Here's how the part is built. I have some questions about the finished solid (model axes, mm). A direction names the side the tool comes from. Coordinates: 2 decimals unless noted, no trailing zeros. Write each loop counter-clockwise with the first axis right and the second up, starting at its lowest first coordinate (ties: lowest second). Pieces come first, ordered by that corner, then holes. Notation, with made-up numbers: (25, 59) -> (33, 59) arc R24 cw to (33, 96) -> close; hole circle Ø11 at (57, -20.75). An arc over 180 degrees is marked (long way). Put each result on its own line as item: value. Start each with the question number.
Item 1: I need wall thicknesses on line 1 (Y direction, x = -11.5, z = 7); line 2 (X direction, y = -11.5, z = 4.5). Which ranges of each line are inside material? Lowest first, please. Write a range as [from, to].
Item 2: I want a section at A-A, the plane z = 9. List the corners of the cut face in (x, y) for me, then the cut area to 4 significant figures.
Item 3: I want a section at B-B, the plane x = 9.5. List the corners of the cut face in (y, z) for me.
Item 4: On a 3-axis mill with a long thin cutter (end or side, diameter ignored), from which of +Z, -Z, +X, -X, +Y, -Y can I reach the whole of each face in a straight line? I mean faces 1 (the face through (15.5, 11.5, 4.2)), 2 (the face through (0, 14, 1)), 3 (the face through (0, -14, 1)). Say none if no direction works.
Item 5: I want a section at C-C, the plane y = 11.5. List the corners of the cut face in (x, z) for me, then the cut area to 3 significant figures.
Item 6: For pin 1 (1.8 mm diameter, centred on x = -0.5, y = 15, fed in from +Z); pin 2 (2.5 mm diameter, centred on x = -5.5, z = 3, fed in from +Y); pin 3 (4 mm diameter, centred on x = 3, z = 1.5, fed in from +Y), each with a flat end and sliding along its axis, tell me the tip position at first contact or that it passes through.
Item 7: I want a section at D-D, the plane x = -5. List the corners of the cut face in (y, z) for me.
from build123d import *

# Parameters (mm, degrees)
F0_W        = 5
F0_H        = 6
F1_DEPTH    = 9.5
F2_DEPTH    = 1
F3_T1_DEPTH = 1
F3_T3_DEPTH = 16
F4_SIZE     = 1


# Not quite as in the source:
# - a fillet or chamfer that OpenCascade refuses, or shapes differently, is made with other operations: its cross-section is extruded or revolved along the edge and cut away or added


with BuildPart() as f1:
    # F0 (on Top) → F1 (new body)
    with BuildSketch(Plane.XY):
        Polygon((16, -12), (16, 12), (2.5, 12), (2.5, 6), (-2.5, 6), (-2.5, 12), (-16, 12), (-16, -12), (-2.5, -12), (-2.5, -6), (2.5, -6), (2.5, -12), align=None)
        with Locations((0, -9)):
            Rectangle(F0_W, F0_H)
        with Locations((0, 9)):
            Rectangle(F0_W, F0_H)
    extrude(amount=F1_DEPTH)

    # F0 (on Top) → F2 (join)
    with BuildSketch(Plane.XY):
        with Locations((0, 15)):
            Rectangle(F0_W, F0_H)
        with Locations((0, -15)):
            Rectangle(F0_W, F0_H)
    extrude(amount=F2_DEPTH)

    # F3: fillet of radius 3 on 8 edges, made by hand

    # F3_s2 → F3_t1 (join)
    with BuildSketch(Plane.XY):
        with BuildLine():
            ThreePointArc((5.5, -12), (3.3786796564, -12.8786796564), (2.5, -15))
            Line((2.5, -15), (2.5, -12))
            Line((2.5, -12), (5.5, -12))
        make_face()
        with BuildLine():
            ThreePointArc((-5.5, -12), (-3.3786796564, -12.8786796564), (-2.5, -15))
            Line((-2.5, -15), (-2.5, -12))
            Line((-2.5, -12), (-5.5, -12))
        make_face()
        with BuildLine():
            ThreePointArc((-5.5, 12), (-3.3786796564, 12.8786796564), (-2.5, 15))
            Line((-2.5, 15), (-2.5, 12))
            Line((-2.5, 12), (-5.5, 12))
        make_face()
        with BuildLine():
            ThreePointArc((5.5, 12), (3.3786796564, 12.8786796564), (2.5, 15))
            Line((2.5, 15), (2.5, 12))
            Line((2.5, 12), (5.5, 12))
        make_face()
    extrude(amount=F3_T1_DEPTH)

    # F3_s4 → F3_t3 (cut)
    with BuildSketch(Plane.XY.offset(-7.5)):
        with BuildLine():
            ThreePointArc((0.5, -18), (-1.6213203436, -17.1213203436), (-2.5, -15))
            Line((-2.5, -15), (-2.5, -18))
            Line((-2.5, -18), (0.5, -18))
        make_face()
        with BuildLine():
            ThreePointArc((2.5, -15), (1.6213203436, -17.1213203436), (-0.5, -18))
            Line((-0.5, -18), (2.5, -18))
            Line((2.5, -18), (2.5, -15))
        make_face()
        with BuildLine():
            ThreePointArc((-2.5, 15), (-1.6213203436, 17.1213203436), (0.5, 18))
            Line((0.5, 18), (-2.5, 18))
            Line((-2.5, 18), (-2.5, 15))
        make_face()
        with BuildLine():
            ThreePointArc((-0.5, 18), (1.6213203436, 17.1213203436), (2.5, 15))
            Line((2.5, 15), (2.5, 18))
            Line((2.5, 18), (-0.5, 18))
        make_face()
    extrude(amount=F3_T3_DEPTH, mode=Mode.SUBTRACT)

    # F4
    f4_edges = [f1.edges().sort_by_distance(p)[0] for p in [
        (-16, 0, 9.5),
        (0, 12, 9.5),
        (0, -12, 9.5),
        (16, 0, 9.5),
        (-16, 12, 4.75),
        (-16, -12, 4.75),
        (16, -12, 4.75),
        (16, 12, 4.75),
    ]]
    chamfer(f4_edges, length=F4_SIZE)


solid = f1.part
Calculated:
1. line 1: y = [-12, 12]
1. line 2: x = [-15.5, 15.5]
2. outline: (-15.5, -11) -> (-15, -11.5) -> (15, -11.5) -> (15.5, -11) -> (15.5, 11) -> (15, 11.5) -> (-15, 11.5) -> (-15.5, 11) -> close
2. area: 712.5 mm2
3. outline: (-12, 0) -> (12, 0) -> (12, 8.5) -> (11, 9.5) -> (-11, 9.5) -> (-12, 8.5) -> close
4. face 1: +Z, -Z, +X, +Y
4. face 2: +Z, +X, -X, +Y
4. face 3: +Z, +X, -X, -Y
5. outline: (-15.5, 0) -> (15.5, 0) -> (15.5, 8.5) -> (15, 9) -> (-15, 9) -> (-15.5, 8.5) -> close
5. area: 279 mm2
6. pin 1: stops at z = 1
6. pin 2: stops at y = 12
6. pin 3: stops at y = 17.56
7. outline: (-12.04, 0) -> (12.04, 0) -> (12.04, 1) -> (12, 1) -> (12, 8.5) -> (11, 9.5) -> (-11, 9.5) -> (-12, 8.5) -> (-12, 1) -> (-12.04, 1) -> close
